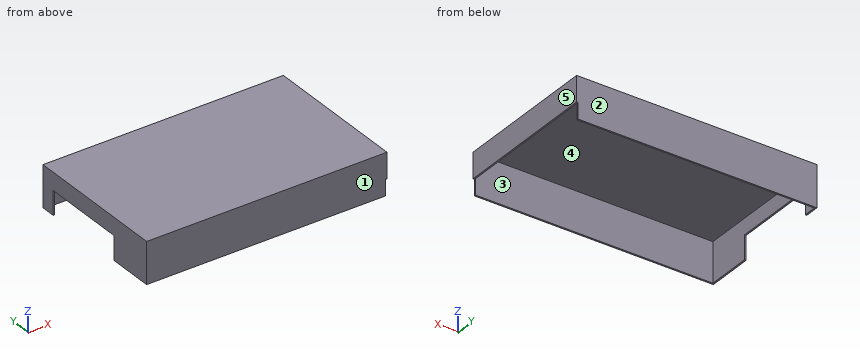
```python
from build123d import *

# Parameters (mm, degrees)
F0_W     = 1
F0_H     = 54
F1_DEPTH = 1
F2_DEPTH = 25
F3_DEPTH = 10
F4_DEPTH = 15


with BuildPart() as f1:
    # F0 (on Top) → F1 (new body)
    with BuildSketch(Plane.XY):
        with Locations((0.5, 56)):
            Rectangle(F0_W, F0_H)
        Polygon((150, 1), (150, 0), (151, 0), (151, 92), (150, 92), (150, 91), align=None)
        Polygon((1, 1), (150, 1), (150, 91), (1, 91), (1, 83), (1, 29), align=None)
        Polygon((0, 92), (0, 83), (1, 83), (1, 91), (150, 91), (150, 92), align=None)
        Polygon((0, 29), (0, 0), (150, 0), (150, 1), (1, 1), (1, 29), align=None)
    extrude(amount=F1_DEPTH)

    # F0 (on Top) → F2 (join)
    with BuildSketch(Plane.XY):
        Polygon((0, 29), (0, 0), (150, 0), (150, 1), (1, 1), (1, 29), align=None)
        Polygon((0, 92), (0, 83), (1, 83), (1, 91), (150, 91), (150, 92), align=None)
    extrude(amount=-F2_DEPTH)

    # F0 (on Top) → F3 (join)
    with BuildSketch(Plane.XY):
        with Locations((0.5, 56)):
            Rectangle(F0_W, F0_H)
    extrude(amount=-F3_DEPTH)

    # F0 (on Top) → F4 (join)
    with BuildSketch(Plane.XY):
        Polygon((150, 1), (150, 0), (151, 0), (151, 92), (150, 92), (150, 91), align=None)
    extrude(amount=-F4_DEPTH)


solid = f1.part
```
Read the model definition and answer for the solid it produces. Units are mm, in the model's axes. Face numbers are marked on the shaded views. A direction names the side the tool comes from. Give positions to 0.01 mm unless a question says otherwise; leave off trailing zeros. Write each loop counter-clockwise with the first axis right and the second up, starting at its lowest first coordinate (ties: lowest second). Pieces come first, ordered by that corner, then holes. Notation, with made-up numbers: (10, 52.25) - (32, 52.25) arc R5 cw to (32, 58.25) - close; hole circle Ø6 at (-37.5, 77.5). An arc over 180 degrees is marked (long way). Write item = value, one per line. Start each with the question number.
Item 1: Find section A-A (z = -21.5). Give the vertices of the cut face in (x, y).
Item 2: Find the intervals of material crossed by probe 1 along X at (y, z) = (88, -9.25); probe 2 along Y at (x, z) = (8, -21); probe 3 along Z at (x, y) = (65, 17), in increasing order. Write a range as [from, to].
Item 3: A tool of negligible diameter and unlimited length cuts with its end or side. For the marked faces 4 and 5, from which of +Z, -Z, +X, -X, +Y, -Y can it reach the whole face along a straight path? Write none if from no direction.
Item 4: Each of these flat-tipped pins is pushed along its axis until it touches: P1, Ø2, axis at x = 103.5, y = 21, coming from the -Z side; P2, Ø5, axis at y = 72.5, z = -10, coming from the -X side; P3, Ø0.5, axis at x = 150.5, y = 36, coming from the -Z side; P4, Ø1.1, axis at y = 0.5, z = -20, coming from the +X side. Where does it stop, or does it pass through?
Item 5: Find section B-B (z = -4). Give the vertices of the cut face in (x, y).
Item 6: The mould has two halves that part along Y. Classify the marked faces 1, 2 and 3: +Y half, -Y half, draft (parallel to the pull), parting line (faces both ways), or undercut.
Item 7: Find section C-C (y = 48). Give the vertices of the cut face in (x, z), then the cut area to 3 significant figures.
Item 8: Find section D-D (x = 65). Give the vertices of the cut face in (y, z).
Response:
q1.outline = (0, 0) - (150, 0) - (150, 1) - (1, 1) - (1, 29) - (0, 29) - close; (0, 83) - (1, 83) - (1, 91) - (150, 91) - (150, 92) - (0, 92) - close
q2.probe_1 = [0, 1], [150, 151]
q2.probe_2 = [0, 1], [91, 92]
q2.probe_3 = [0, 1]
q3.face_4 = -Z
q3.face_5 = +Z, -Z, +X, +Y, -Y
q4.P1 = 0
q4.P2 = 0
q4.P3 = -15
q4.P4 = 150
q5.outline = (0, 0) - (151, 0) - (151, 92) - (0, 92) - close; hole (1, 1) - (150, 1) - (150, 91) - (1, 91) - close
q6.face_1 = -Y half
q6.face_2 = +Y half
q6.face_3 = undercut
q7.outline = (0, -10) - (1, -10) - (1, 0) - (150, 0) - (150, -15) - (151, -15) - (151, 1) - (0, 1) - close
q7.area = 176 mm²
q8.outline = (0, -25) - (1, -25) - (1, 0) - (91, 0) - (91, -25) - (92, -25) - (92, 1) - (0, 1) - close
